Geometry check sheet. Reference: drawing and pictorial views, mm from the part's lowest x, y, z. Give positions to 0.01 mm unless a question says otherwise; leave off trailing zeros. Write each loop counter-clockwise with the first axis right and the second up, starting at its lowest first coordinate (ties: lowest second). Pieces come first, ordered by that corner, then holes. Notation, with made-up numbers: (9.5, 51.5) -> (57.5, 51.5) arc R28 cw to (57.5, 89.5) -> close; hole circle Ø7 at (80, -4.75). An arc over 180 degrees is marked (long way). Use a Markdown table: item, result. Add a question column.
1. Cross-section at A-A (x = 26.5). Enter the section's corners in (y, z).
2. Cross-section at C-C (x = 21.25). Enter the section's corners in (y, z), then the cut area to 3 significant figures.
3. Scan lines: probe 1 along X at (y, z) = (8.75, 0.85); probe 2 along X at (y, z) = (11, 0.65); probe 3 along Y at (x, z) = (26.5, 0.45). Record each from-to range of solid material in increasing order. Write a range as [from, to].
4. Cross-section at D-D (z = 1.3). Count the separate pieces of the cut face and the enclosed holes in it.
5. Cross-section at B-B (y = 21.5). Enter the section's corners in (x, z).
6. Gauge pin test, flat end, axial feed: P1, Ø1.9, axis at x = 26.5, y = 21.5, coming from the +Z side. Record the tip position at first contact, or that the pin passes through.
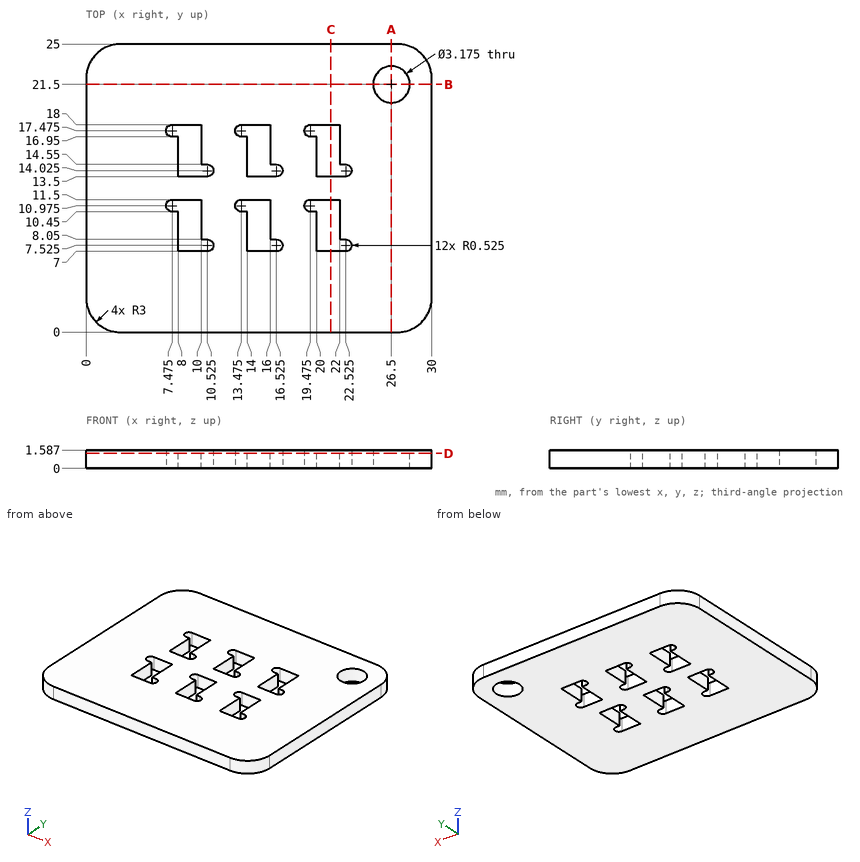
Worked answers:
| question | item | result |
|---|---|---|
| 1 | outline | (0, 0) -> (19.91, 0) -> (19.91, 1.59) -> (0, 1.59) -> close; (23.09, 0) -> (25, 0) -> (25, 1.59) -> (23.09, 1.59) -> close |
| 2 | outline | (0, 0) -> (7, 0) -> (7, 1.59) -> (0, 1.59) -> close; (11.5, 0) -> (13.5, 0) -> (13.5, 1.59) -> (11.5, 1.59) -> close; (18, 0) -> (25, 0) -> (25, 1.59) -> (18, 1.59) -> close |
| 2 | area | 25.4 mm² |
| 3 | probe 1 | x = [0, 8], [10, 14], [16, 20], [22, 30] |
| 3 | probe 2 | x = [0, 6.95], [10, 12.95], [16, 18.95], [22, 30] |
| 3 | probe 3 | y = [0, 19.91], [23.09, 25] |
| 4 | separate pieces | 1 |
| 4 | enclosed holes | 7 |
| 5 | outline | (0, 0) -> (24.91, 0) -> (24.91, 1.59) -> (0, 1.59) -> close; (28.09, 0) -> (30, 0) -> (30, 1.59) -> (28.09, 1.59) -> close |
| 6 | P1 | passes through |
